Autodesk Inventor part; units mm, degrees
ref_plane "YZ Plane" through (0, 0, 0) normal (1, 0, 0) x (0, 1, 0)
ref_plane "XZ Plane" through (0, 0, 0) normal (0, 1, 0) x (-1, 0, 0)
ref_plane "XY Plane" through (0, 0, 0) normal (0, 0, 1) x (1, 0, 0)
sketch "Sketch2" plane through (0, 0, 0) normal (0, 1, 0) x (-1, 0, 0)
  line L0 (4.5, 4) -> (-4.5, 4)
  line L1 (4.5, 4) -> (4.5, 7.5)
  line L2 (4.5, 7.5) -> (3.5, 7.5)
  line L3 (3.5, 7.5) -> (3.5, 5)
  line L4 (3.5, 5) -> (-4.5, 5)
  line L5 (-4.5, 5) -> (-4.5, 4)
  line L6 (4.5, 0) -> (-4.5, 0)
  point P0 (0, 0)
  point P1 (0, 0)
  dimension "d1" = 9
  dimension "d2" = 1
  dimension "d3" = 1
  dimension "d4" = 3.5
  dimension "d5" = 8
revolve "Revolution1" add sketch "Sketch2" angle 360 about axis through (-4.5, 0, 0) along (1, 0, 0)
fillet "Fillet1" radius 1 1 edges at (-4.5, 0, -4)
chamfer "Chamfer1" distance 0.5 angle 45 1 edges at (4.5, 0, -4)
chamfer "Chamfer2" distance 0.8 distance2 0.3 1 edges at (4.5, 0, -5) measured on face at (1.8333, 0.8021, 4.9353)
equation "\"d3\" = d2"
properties part number "DU BUSH" material "BC"
The model under review builds one solid part; all positions refer to its coordinate system, in mm. A direction names the side the tool comes from. Give positions to 0.01 mm unless a question says otherwise; leave off trailing zeros. Write each loop counter-clockwise with the first axis right and the second up, starting at its lowest first coordinate (ties: lowest second). Pieces come first, ordered by that corner, then holes.
1. Add section A-A, the plane z = 0. Write out the cut boundary in (x, y).
2. Draft analysis for pull direction Y (two halves, no side actions). For faces 3 (the cylindrical face through (0.303, 3.905, -0.867)), 4 (the flat face through (-4.5, 5, 2)), 5 (the cylindrical face through (0.15, 4.88, -1.08)), state which applies: +Y half, -Y half, draft (parallel to the pull), parting line (faces both ways), or undercut.
3. For P1, Ø1.5, axis at x = -2.5, z = -1.5, coming from the +Y side; P2, Ø5, axis at x = -0.5, z = 4, coming from the -Y side; P3, Ø2, axis at x = -3, y = -2, coming from the -Z side, all flat-tipped, find the tip position at first contact; note any pin that passes through.
4. Wall thickness on L1, parallel to Y at x = 2.25, z = 0; L2, parallel to X at y = 5.25, z = -1.25: over which ranges is each line inside the solid? List them lowest first.
5. Tool access review of faces 1 (the cylindrical face through (-3.993, -0.33, -7.493)), 2 (the flat face through (-3.5, 5, 2)): name each direction out of +Z, -Z, +X, -X, +Y, -Y from which nothing blocks a thin tool from reaching the whole face with its end or side.
6. Add section C-C, the plane x = 2.75. Write out the cut boundary in (y, z), plus the area to 3 significant figures.
Worked answers:
1. outline: (-4.5, -7.5) - (-3.5, -7.5) - (-3.5, -5) - (3.7, -5) - (4.5, -4.7) - (4.5, -4.5) - (4, -4) - (-3.5, -4) arc R1 ccw to (-4.5, -5) - close; (-4.5, 5) arc R1 ccw to (-3.5, 4) - (4, 4) - (4.5, 4.5) - (4.5, 4.7) - (3.7, 5) - (-3.5, 5) - (-3.5, 7.5) - (-4.5, 7.5) - close
2. face 3: undercut
2. face 4: draft
2. face 5: parting line
3. P1: stops at y = 4.94
3. P2: stops at y = -4.77
3. P3: stops at z = -7.41
4. L1: y = -5 to -4, 4 to 5
4. L2: x = -4.5 to -3.5
5. face 1: +X, -X
5. face 2: +X
6. outline: circle Ø10 at (0, 0); hole circle Ø8 at (0, 0)
6. area: 28.3 mm2
